```python
from build123d import *

# Parameters (mm, degrees)
F4_DEPTH = 2.5
F6_D     = 6.6
F6_DEPTH = 20
F6_TIP   = 1.9828400428


with BuildPart() as f1:
    # F0 (on Front) → F1 (revolve)
    with BuildSketch(Plane.XZ):
        Polygon((0, 20), (0, 0), (74, 0), (74, 6), (32.5, 6), (32.5, 7.5), (20.5, 7.5), (20.5, 7.15), (19.4, 7.15), (19.4, 7.5), (4, 7.5), (4, 20), align=None)
    revolve(axis=Axis((37, 0, 0), (-1, 0, 0)))

    # F3 (on offset) → F4 (cut)
    with BuildSketch(Plane.XY.offset(6)):
        with BuildLine():
            ThreePointArc((42, 2), (40, 0), (42, -2))
            Line((42, -2), (64, -2))
            ThreePointArc((64, -2), (66, 0), (64, 2))
            Line((64, 2), (42, 2))
        make_face()
    extrude(amount=-F4_DEPTH, mode=Mode.SUBTRACT)

    # F6
    with Locations(Plane(origin=(0, 0, 0), x_dir=(0, -1, 0), z_dir=(-1, 0, 0))):
        with Locations((0, 0)):
            Hole(F6_D / 2, depth=F6_DEPTH)
            with Locations((0, 0, -(F6_DEPTH + F6_TIP / 2))):  # 118° drill point
                Cone(0, F6_D / 2, F6_TIP, mode=Mode.SUBTRACT)


solid = f1.part
```
CAD build for the part. Positions are in the model's coordinates, mm. A direction names the side the tool comes from. Round coordinates to 2 decimals unless told otherwise and drop trailing zeros. Order: outer loops, then holes, each group sorted by start corner. A loop starts at its lowest first (then second) coordinate and runs counter-clockwise, first axis right, second up. Notation, with made-up numbers: (-17.5, 50) - (-12.5, 50) arc R4 cw to (-12.5, 56) - close; hole circle Ø6 at (34, 54). An arc over 180 degrees is marked (long way). Answer as CSV lines item,"result". Start each with the question number.
1. Saw through at C-C, the plane z = 9. Write the cut outline in (x, y), and give its area (3 significant figures).
2. Pin check, flat tips, straight feed: pin 1 (12 mm diameter, centred on y = -5.5, z = -14.5, fed in from +X); pin 2 (1.5 mm diameter, centred on x = 30, y = -4.5, fed in from +Z); pin 3 (0.6 mm diameter, centred on x = 55, z = 4.5, fed in from +Y). Stop position of each tip, or through.
3. Pull direction Z, two halves, no side cores. Call faces 1 (the face through (74, 0, 0)), 2 (the face through (10.14, -2.43, 2.23)), 3 (the face through (53, 0, 3.5)), 4 (the face through (11.592, 0.33, -7.493)): +Z half, -Z half, draft (parallel to the pull), parting line (faces both ways), or undercut.
4. Tool access for faces 5 (the face through (40, 0, 5)), 6 (the face through (19.94, 7.09, -0.93)), 7 (the face through (26.416, 0.33, -7.493)): list every direction of +Z, -Z, +X, -X, +Y, -Y with a clear straight run to the whole face (end or side of a thin tool).
5. Saw through at B-B, the plane x = 27. Write the cut outline in (y, z), and give its area (3 significant figures).
6. Saw through at A-A, the plane y = -12. Write the cut outline in (x, z), and give its area (3 significant figures).
7. Drill centre lines: L1, parallel to Y at x = 13.75, z = 0; L2, parallel to X at y = -8.5, z = -5; L3, parallel to Z at x = 6.5, y = 3. Where is each one in solid material? Low to high. Write a range as [from, to].
Model answer:
1,outline,"(0, -17.86) - (4, -17.86) - (4, 17.86) - (0, 17.86) - close"
1,area,"143 mm²"
2,pin 1,"stops at x = 4"
2,pin 2,"stops at z = 6.5"
2,pin 3,"stops at y = 4.28"
3,face 1,"draft"
3,face 2,"undercut"
3,face 3,"+Z half"
3,face 4,"parting line"
4,face 5,"+Z"
4,face 6,"none"
4,face 7,"+X"
5,outline,"circle Ø15 at (0, 0)"
5,area,"177 mm²"
6,outline,"(0, -16) - (4, -16) - (4, 16) - (0, 16) - close"
6,area,"128 mm²"
7,L1,"y = [-7.5, -3.3], [3.3, 7.5]"
7,L2,"x = [0, 4]"
7,L3,"z = [-6.87, -1.37], [1.37, 6.87]"
